Check sheet for the modelled part. Datum: model origin and axes. Units: mm. Round coordinates to 2 decimals unless told otherwise and drop trailing zeros. Loops run counter-clockwise (first coordinate to the right, second up) from the corner with the lowest first, then second, coordinate; pieces in that order, holes last. Notation, with made-up numbers: (-7, 9) - (10, 9) arc R12 ccw to (10, 15) - close; hole circle Ø8 at (82.25, -17). An arc over 180 degrees is marked (long way). Answer in a Markdown table with one row per item. Add a question column.
(1) Cross-section at B-B on z = 1.65. Enter the section's corners in (x, y) (3 decimals).
(2) Thickness scan on line 1 along Y through (x, z) = (0, 1.7); line 2 along X through (y, z) = (0.95, 0.2); line 3 along X through (y, z) = (0.4, 1.8). Record the ranges inside material, lowest first.
(3) Cross-section at A-A on x = 0. Enter the section's corners in (y, z).
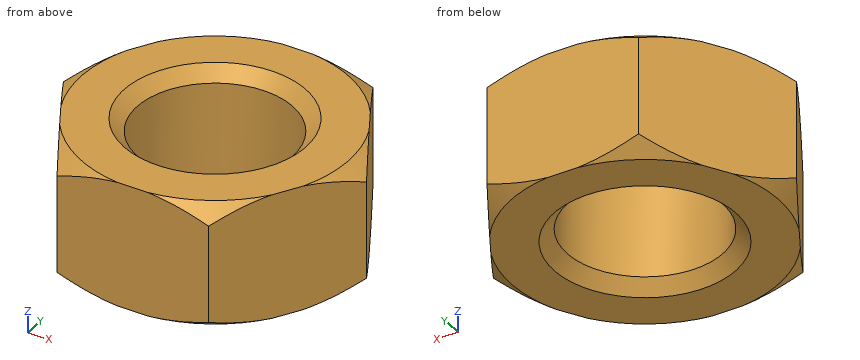
from build123d import *

# Parameters (mm, degrees)
SKETCH1_R           = 1.5
BOSS_EXTRUDE1_DEPTH = 2.4
CHAMFER1_SIZE       = 0.25


with BuildPart() as part:
    # Sketch1 → Boss-Extrude1 (new body)
    with BuildSketch(Plane.XY):
        Polygon((2.95, 0), (1.475, 2.554774941), (-1.475, 2.554774941), (-2.95, 0), (-1.475, -2.554774941), (1.475, -2.554774941), align=None)
        Circle(SKETCH1_R, mode=Mode.SUBTRACT)
    extrude(amount=BOSS_EXTRUDE1_DEPTH)

    # Chamfer1
    chamfer1_edges = [part.edges().sort_by_distance(p)[0] for p in [
        (-1.5, 0, 0),
        (-1.5, 0, 2.4),
    ]]
    chamfer(chamfer1_edges, length=CHAMFER1_SIZE)

    # Sketch2 → Cut-Revolve1 (revolve, cut)
    with BuildSketch(Plane(origin=(0, 0, 0), x_dir=(1, 0, 0), z_dir=(0, 1, 0))):
        Polygon((-1, -2.45), (-2.5, -2.45), (-3.132844885, -2.006877241), (-3.132844885, -0.393122759), (-2.5, 0.05), (-1, 0.05), (-1, 1.98132807), (-7.750900281, 1.98132807), (-7.750900281, -6.982873217), (-1, -6.982873217), align=None)
    revolve(axis=Axis((0, 0, 2.45), (0, 0, -1)), mode=Mode.SUBTRACT)


solid = part.part
Answers:
| question | item | result |
|---|---|---|
| 1 | outline | (-2.95, 0) - (-1.475, -2.555) - (1.475, -2.555) - (2.95, 0) - (1.475, 2.555) - (-1.475, 2.555) - close; hole circle Ø3 at (0, 0) |
| 2 | line 1 | y = -2.55 to -1.5, 1.5 to 2.55 |
| 2 | line 2 | x = -2.4 to -1.22, 1.22 to 2.4 |
| 2 | line 3 | x = -2.72 to -1.45, 1.45 to 2.72 |
| 3 | outline | (-2.55, 0) - (-1.75, 0) - (-1.5, 0.25) - (-1.5, 2.15) - (-1.75, 2.4) - (-2.55, 2.4) - close; (1.5, 0.25) - (1.75, 0) - (2.55, 0) - (2.55, 2.4) - (1.75, 2.4) - (1.5, 2.15) - close |
